Read the model definition and answer for the solid it produces. Units are mm, in the model's axes. A direction names the side the tool comes from. Coordinates: 2 decimals unless noted, no trailing zeros. Loops run counter-clockwise (first coordinate to the right, second up) from the corner with the lowest first, then second, coordinate; pieces in that order, holes last. Notation, with made-up numbers: M -28.5,59 L 22.5,59 A20 ccw 22.5,67 Z; hole C 48,-14 d11. An arc over 180 degrees is marked long. One line per item, written item: value. Start each with the question number.
```python
from build123d import *

# Parameters (mm, degrees)
SKETCH1_W           = 15
SKETCH1_H           = 30
BOSS_EXTRUDE1_DEPTH = 2
SKETCH2_R           = 3.5
BOSS_EXTRUDE2_DEPTH = 15
CUT_EXTRUDE1_REACH  = 83.672
SKETCH3_R           = 1.75
SKETCH4_R           = 3
SKETCH4_R_2         = 1.75
BOSS_EXTRUDE3_DEPTH = 5
FILLET1_R           = 5
FILLET2_R           = 3.5


with BuildPart() as part:
    # Sketch1 → Boss-Extrude1 (new body)
    with BuildSketch(Plane(origin=(0, 0, 0), x_dir=(1, 0, 0), z_dir=(0, 1, 0))):
        Polygon((-75, 27.5), (-75, -27.5), (-10, -27.5), (-10, -20), (10, -20), (10, -27.5), (75, -27.5), (75, 27.5), (10, 27.5), (10, 20), (-10, 20), (-10, 27.5), align=None)
        with Locations((-50.25, 2.25)):
            Rectangle(SKETCH1_W, SKETCH1_H, mode=Mode.SUBTRACT)
    extrude(amount=BOSS_EXTRUDE1_DEPTH)

    # Sketch2 → Boss-Extrude2 (add)
    with BuildSketch(Plane(origin=(0, 2, 0), x_dir=(1, 0, 0), z_dir=(0, 1, 0))):
        with Locations(Location((-67.75, -19.5, 0), (0, 0, 270))):
            Circle(SKETCH2_R)
        with Locations(Location((-67.75, 24, 0), (0, 0, 90))):
            Circle(SKETCH2_R)
        with Locations(Location((67.75, 24, 0), (0, 0, 90))):
            Circle(SKETCH2_R)
        with Locations(Location((67.75, -19.5, 0), (0, 0, 270))):
            Circle(SKETCH2_R)
    extrude(amount=BOSS_EXTRUDE2_DEPTH)

    # Sketch3 → Cut-Extrude1 (cut, up to next)
    with BuildSketch(Plane(origin=(0, 17, 0), x_dir=(1, 0, 0), z_dir=(0, 1, 0)), mode=Mode.PRIVATE) as cut_extrude1_sk1:
        with Locations(Location((-67.75, -19.5, 0), (0, 0, 270))):
            Circle(SKETCH3_R)
    cut_extrude1_tool1 = extrude(cut_extrude1_sk1.sketch, amount=-CUT_EXTRUDE1_REACH, mode=Mode.PRIVATE) & part.part
    # Sketch3 → Cut-Extrude1 (cut, up to next)
    with BuildSketch(Plane(origin=(0, 17, 0), x_dir=(1, 0, 0), z_dir=(0, 1, 0)), mode=Mode.PRIVATE) as cut_extrude1_sk2:
        with Locations(Location((-67.75, 24, 0), (0, 0, 270))):
            Circle(SKETCH3_R)
    cut_extrude1_tool2 = extrude(cut_extrude1_sk2.sketch, amount=-CUT_EXTRUDE1_REACH, mode=Mode.PRIVATE) & part.part
    # Sketch3 → Cut-Extrude1 (cut, up to next)
    with BuildSketch(Plane(origin=(0, 17, 0), x_dir=(1, 0, 0), z_dir=(0, 1, 0)), mode=Mode.PRIVATE) as cut_extrude1_sk3:
        with Locations(Location((67.75, 24, 0), (0, 0, 270))):
            Circle(SKETCH3_R)
    cut_extrude1_tool3 = extrude(cut_extrude1_sk3.sketch, amount=-CUT_EXTRUDE1_REACH, mode=Mode.PRIVATE) & part.part
    # Sketch3 → Cut-Extrude1 (cut, up to next)
    with BuildSketch(Plane(origin=(0, 17, 0), x_dir=(1, 0, 0), z_dir=(0, 1, 0)), mode=Mode.PRIVATE) as cut_extrude1_sk4:
        with Locations(Location((67.75, -19.5, 0), (0, 0, 270))):
            Circle(SKETCH3_R)
    cut_extrude1_tool4 = extrude(cut_extrude1_sk4.sketch, amount=-CUT_EXTRUDE1_REACH, mode=Mode.PRIVATE) & part.part
    add(cut_extrude1_tool1.solids().sort_by_distance((-67.75, 17, 19.5))[0], mode=Mode.SUBTRACT)
    add(cut_extrude1_tool2.solids().sort_by_distance((-67.75, 17, -24))[0], mode=Mode.SUBTRACT)
    add(cut_extrude1_tool3.solids().sort_by_distance((67.75, 17, -24))[0], mode=Mode.SUBTRACT)
    add(cut_extrude1_tool4.solids().sort_by_distance((67.75, 17, 19.5))[0], mode=Mode.SUBTRACT)

    # Sketch4 → Boss-Extrude3 (add)
    # profile 1 of 2: a face of its own
    with BuildSketch(Plane(origin=(0, 2, 0), x_dir=(1, 0, 0), z_dir=(0, 1, 0))):
        with Locations(Location((-3.66, 2.25, 0), (0, 0, 270))):
            Circle(SKETCH4_R)
        with Locations(Location((-3.66, 2.25, 0), (0, 0, 270))):
            Circle(SKETCH4_R_2, mode=Mode.SUBTRACT)
    # profile 2 of 2: a face of its own
    with BuildSketch(Plane(origin=(0, 2, 0), x_dir=(1, 0, 0), z_dir=(0, 1, 0))):
        with Locations(Location((70, 2.25, 0), (0, 0, 270))):
            Circle(SKETCH4_R)
        with Locations(Location((70, 2.25, 0), (0, 0, 270))):
            Circle(SKETCH4_R_2, mode=Mode.SUBTRACT)
    extrude(amount=BOSS_EXTRUDE3_DEPTH)

    # Fillet1
    fillet1_edges = [part.edges().sort_by_distance(p)[0] for p in [
        (-57.75, 1, -17.25),
        (-57.75, 1, 12.75),
        (-42.75, 1, 12.75),
        (-42.75, 1, -17.25),
        (-75, 1, 27.5),
        (-75, 1, -27.5),
        (75, 1, -27.5),
        (75, 1, 27.5),
    ]]
    fillet(fillet1_edges, radius=FILLET1_R)

    # Fillet2
    fillet2_edges = [part.edges().sort_by_distance(p)[0] for p in [
        (10, 1, 20),
        (-10, 1, 20),
        (-10, 1, 27.5),
        (-10, 1, -27.5),
        (-10, 1, -20),
        (10, 1, -20),
        (10, 1, -27.5),
        (10, 1, 27.5),
    ]]
    fillet(fillet2_edges, radius=FILLET2_R)


solid = part.part
```
1) Section D-D (x = 2) is taken. Determine the outline of the cut face in (y, z), then the cut area to 3 significant figures.
2) Section C-C (x = -55) is taken. Determine the outline of the cut face in (y, z), then the cut area to 3 significant figures.
3) A tool of negligible diameter and unlimited length cuts with its end or side. For faces 1 (the face through (-1.63, 4.46, -4.46)), 2 (the face through (-11.05, 1.01, -26.5)), 3 (the face through (11, 1.01, 26.45)), 4 (the face through (-56.25, 1.01, 11.32)), from which of +Z, -Z, +X, -X, +Y, -Y can it reach the whole face along a straight path? Write none if from no direction.
4) For a pull along X with two mould halves and no side action, classify faces 5 (the face through (-44.18, 1.01, -15.75)), 6 (the face through (-66.7, 9.4, 22.84)), 7 (the face through (-6, 7, -2)), 8 (the face through (-73.57, 1.01, -26)) as released by +X, released by -X, zero draft, split by the parting line, or undercut.
5) Flat-ended cylindrical pins translate along their axes: pin 1 (3 mm diameter, centred on x = 5.5, y = 3, fed in from +Z); pin 2 (8 mm diameter, centred on x = 48.5, z = -14.5, fed in from +Y); pin 3 (8 mm diameter, centred on y = 14.5, z = 16, fed in from +X). Find the tip coordinate at first contact, or state that the pin passes through.
6) Section B-B (y = 14.25) is taken. Determine the outline of the cut face in (x, z), then the cut area to 3 significant figures.
7) Consider line 1 along X through (y, z) = (7, -24); line 2 along X through (y, z) = (15.75, -25); line 3 along Y through (x, z) = (-42.5, 13.5). Determine where each line is inside the solid, lowest interval first.
8) Section A-A (z = -2.25) is taken. Determine the outline of the cut face in (x, y), then the cut area to 3 significant figures.
Results found:
1. outline: M 0,-20 L 2,-20 L 2,20 L 0,20 Z
1. area: 80.0 mm²
2. outline: M 0,-27.5 L 2,-27.5 L 2,-16.72 L 0,-16.72 Z; M 0,12.22 L 2,12.22 L 2,27.5 L 0,27.5 Z
2. area: 52.1 mm²
3. face 1: +Y
3. face 2: -Z, +Y, -Y
3. face 3: +Z, +Y, -Y
3. face 4: +Y, -Y
4. face 5: undercut
4. face 6: undercut
4. face 7: zero draft
4. face 8: released by -X
5. pin 1: stops at z = 20
5. pin 2: stops at y = 2
5. pin 3: stops at x = 71.25
6. outline: C -67.75,-24 d7; C -67.75,19.5 d7; C 67.75,-24 d7; C 67.75,19.5 d7; hole C -67.75,-24 d3.5; hole C -67.75,19.5 d3.5; hole C 67.75,-24 d3.5; hole C 67.75,19.5 d3.5
6. area: 115 mm²
7. line 1: x = -71.25 to -69.5, -66 to -64.25, 64.25 to 66, 69.5 to 71.25
7. line 2: x = -71.1 to -69.19, -66.31 to -64.4, 64.4 to 66.31, 69.19 to 71.1
7. line 3: y = 0 to 2
8. outline: M -75,0 L -57.75,0 L -57.75,2 L -75,2 Z; M -42.75,0 L 75,0 L 75,2 L 73,2 L 73,7 L 71.75,7 L 71.75,2 L 68.25,2 L 68.25,7 L 67,7 L 67,2 L -0.66,2 L -0.66,7 L -1.91,7 L -1.91,2 L -5.41,2 L -5.41,7 L -6.66,7 L -6.66,2 L -42.75,2 Z
8. area: 295 mm²
